CAD build for the part. Positions are in the model's coordinates, mm. A direction names the side the tool comes from. Coordinates: 2 decimals unless noted, no trailing zeros. Order: outer loops, then holes, each group sorted by start corner. A loop starts at its lowest first (then second) coordinate and runs counter-clockwise, first axis right, second up. Notation, with made-up numbers: (-30, 40) - (27, 40) arc R19 cw to (27, 65) - close; hole circle Ø10 at (-14.5, 75). An arc over 180 degrees is marked (long way). Write each question's results on one line, items separated by ' | '. Start each with the question number.
Q1. Pin check, flat tips, straight feed: P1, Ø1.5, axis at y = 54.5, z = -68.5, coming from the -X side; P2, Ø12, axis at x = -64.5, y = 88.5, coming from the -Z side; P3, Ø1, axis at x = -57.5, z = 78.5, coming from the -Y side. Stop position of each tip, or through.
Q2. Which spindle directions (+Z, -Z, +X, -X, +Y, -Y) get a long thin tool onto all of the face, cutting with end or side? Do faces 4 (the flat face through (-2, 0, -23)), 5 (the flat face through (-1, 75, 87)). Say none if no direction does.
Q3. Pull direction X, two halves, no side cores. Call faces 1 (the flat face through (-1, 37, 52.98)), 2 (the cylindrical face through (-18.23, 73.95, -138.81)), 3 (the flat face through (-2, 150, -2)): released by +X, released by -X, zero draft, split by the parting line, or undercut.
Q4. Band-saw the part on B-B, the plane x = 0. Write the cut outline in (y, z), then the cut area to 3 significant figures.
Q5. Band-saw the part on D-D, the plane x = 48. Write the cut outline in (y, z), then the cut area to 3 significant figures.
Q6. Wall check: probe 1 along Y at (x, z) = (-68, 73); probe 2 along X at (y, z) = (36, 75); probe 3 along X at (y, z) = (126.5, -1.5). Give the ranges that are in metal, low to high.
Q7. Band-saw the part on A-A, the plane z = 89. Write the cut outline in (x, y).
Q8. Band-saw the part on C-C, the plane y = 139. Write the cut outline in (x, z).
```python
from build123d import *

# Parameters (mm, degrees)
SKETCH1_R           = 140
BOSS_EXTRUDE1_DEPTH = 150
CUT_EXTRUDE1_DEPTH  = 75


with BuildPart() as part:
    # Sketch1 → Boss-Extrude1 (new body)
    with BuildSketch(Plane(origin=(0, 0, 0), x_dir=(1, 0, 0), z_dir=(0, 1, 0))):
        Circle(SKETCH1_R)
    extrude(amount=BOSS_EXTRUDE1_DEPTH)

    # Sketch2 → Cut-Extrude1 (cut)
    with BuildSketch(Plane.XZ):
        with BuildLine():
            Line((-100, 97.979589711), (-100, 52.979589711))
            Line((-100, 52.979589711), (100, 52.979589711))
            Line((100, 52.979589711), (100, 97.979589711))
            ThreePointArc((100, 97.979589711), (0, 140), (-100, 97.979589711))
        make_face()
    extrude(amount=-CUT_EXTRUDE1_DEPTH, mode=Mode.SUBTRACT)


solid = part.part
```
Results below:
1) P1: stops at x = -122.52 | P2: stops at z = -127.19 | P3: stops at y = 75
2) face 4: +Z, -Z, +X, -X, -Y | face 5: +Z, -Y
3) face 1: undercut | face 2: split by the parting line | face 3: zero draft
4) outline: (0, -140) - (150, -140) - (150, 140) - (75, 140) - (75, 52.98) - (0, 52.98) - close | area: 35,500 mm²
5) outline: (0, -131.51) - (150, -131.51) - (150, 131.51) - (75, 131.51) - (75, 52.98) - (0, 52.98) - close | area: 33,600 mm²
6) probe 1: y = 75 to 150 | probe 2: x = -118.22 to -100, 100 to 118.22 | probe 3: x = -139.99 to 139.99
7) outline: (-108.07, 0) - (-100, 0) - (-100, 75) - (100, 75) - (100, 0) - (108.07, 0) - (108.07, 150) - (-108.07, 150) - close
8) outline: circle Ø280 at (0, 0)
